Source: three-view drawing plus pictorial views. Frame: mm from the lowest corner of the part. Coordinates: 2 decimals unless noted, no trailing zeros. Order: outer loops, then holes, each group sorted by start corner. A loop starts at its lowest first (then second) coordinate and runs counter-clockwise, first axis right, second up. Notation, with made-up numbers: M -33,3 L -12,3 A21 cw -12,18 Z; hole C 76,38 d10. An arc over 180 degrees is marked long. One line per question, with ' | ' between items.
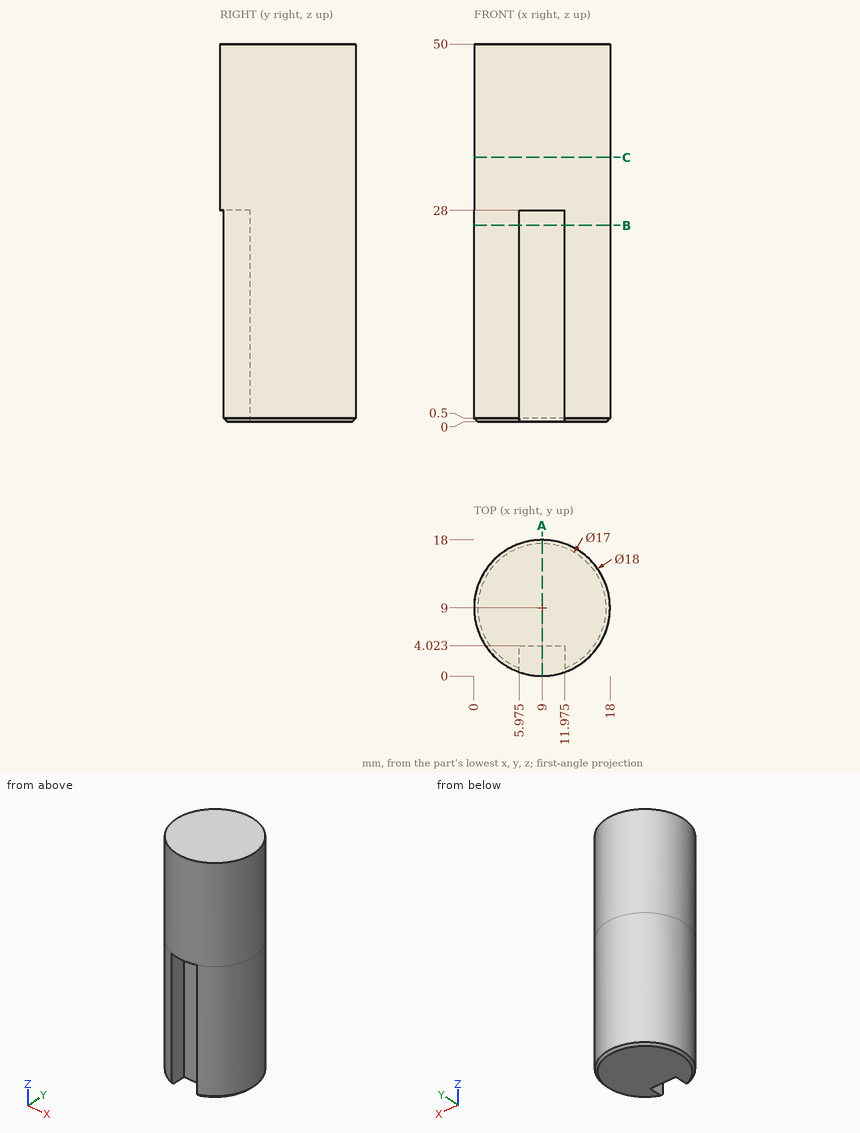
1. Section C-C, the plane z = 35. Output: boundary loops of the cut face in (x, y) (1 decimal).
Response values:
outline: C 9,9 d18
2. Section B-B, the plane z = 26. Output: boundary loops of the cut face in (x, y) (1 decimal), and give its area (3 significant figures).
Response values:
outline: M 6,0.5 L 6,4 L 12,4 L 12,0.5 A9 ccw long Z | area: 231 mm^2
3. Material intervals for line 1 (Z direction, x = 11.5, y = 3.5); line 2 (Y direction, x = 9, z = 19.5); line 3 (Y direction, x = 9.75, z = 34.5), sorted ascending. Write a range as [from, to].
Response values:
line 1: z = [28, 50] | line 2: y = [4.02, 18] | line 3: y = [0.03, 17.97]
4. Section A-A, the plane x = 9. Output: boundary loops of the cut face in (y, z), and give its area (3 significant figures).
Response values:
outline: M 0,28 L 4.02,28 L 4.02,0 L 17.5,0 L 18,0.5 L 18,50 L 0,50 Z | area: 787 mm^2
5. Pin query (flat end, axial travel): P1, Ø1.8, axis at y = 3, z = 7.5, coming from the +X side (1 decimal); P2, Ø1.5, axis at x = 11, y = 2, coming from the -Z side; P3, Ø4, axis at y = 2, z = 11.5, coming from the -X side. Return the tip coordinate at first contact, or that it passes through.
Response values:
P1: stops at x = 16.4 | P2: stops at z = 28 | P3: stops at x = 1.52
